Check sheet for the drawn part. Datum: minimum x, y, z corner. Units: mm. A direction names the side the tool comes from. Give positions to 0.01 mm unless a question says otherwise; leave off trailing zeros. Loops run counter-clockwise (first coordinate to the right, second up) from the corner with the lowest first, then second, coordinate; pieces in that order, holes last.
1. Cross-section at D-D, the plane x = 5.5. Record the cut outline in (y, z).
2. Material ranges on L1, parallel to X at y = 15.1, z = 1.5; L2, parallel to Y at x = 17, z = 4.25; L3, parallel to Z at x = 22, y = 15.25 (1 decimal), recorded low to high.
3. Tool access check on the marked faces 4, 5 and 6. Record the directions out of +Z, -Z, +X, -X, +Y, -Y that give a thin tool (end or side, any length) a straight path to the whole face; none if there is none.
4. Cross-section at B-B, the plane z = 1.5. Record the cut outline in (x, y).
5. Cross-section at A-A, the plane x = 23. Record the cut outline in (y, z).
6. Release check for a two-part mould opening along X. For the marked faces 1, 2 and 3 record: +X half, -X half, draft (parallel to the pull), parting line (faces both ways), or undercut.
7. Cross-section at C-C, the plane z = 7. Record the cut outline in (x, y).
8. Go/stop test with flat-tipped pins: pin 1 Ø3 at (x, y) = (10.5, 3.5) entering from -Z; pin 2 Ø4 at (x, z) = (19, 6.5) entering from -Y; pin 3 Ø3 at (y, z) = (3, 3) entering from -X. Record where each tip stops, or that it passes through.
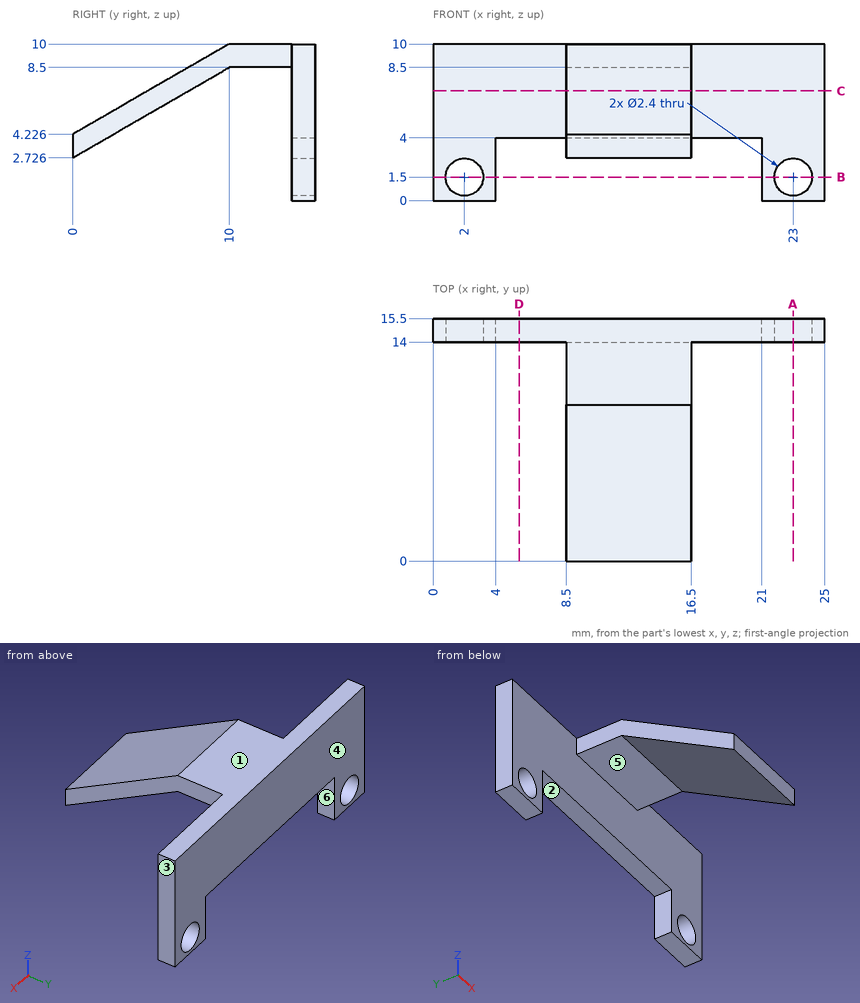
Result:
1. outline: (14, 4) - (15.5, 4) - (15.5, 10) - (14, 10) - close
2. L1: x = 0 to 0.8, 3.2 to 4, 21 to 21.8, 24.2 to 25
2. L2: y = 14 to 15.5
2. L3: z = 0 to 0.8, 2.2 to 10
3. face 4: +Z, -Z, +X, -X, +Y
3. face 5: -Z, +X, -X
3. face 6: -Z, +Y, -Y
4. outline: (0, 14) - (0.8, 14) - (0.8, 15.5) - (0, 15.5) - close; (3.2, 14) - (4, 14) - (4, 15.5) - (3.2, 15.5) - close; (21, 14) - (21.8, 14) - (21.8, 15.5) - (21, 15.5) - close; (24.2, 14) - (25, 14) - (25, 15.5) - (24.2, 15.5) - close
5. outline: (14, 0) - (15.5, 0) - (15.5, 0.3) - (14, 0.3) - close; (14, 2.7) - (15.5, 2.7) - (15.5, 10) - (14, 10) - close
6. face 1: draft
6. face 2: undercut
6. face 3: +X half
7. outline: (0, 14) - (25, 14) - (25, 15.5) - (0, 15.5) - close; (8.5, 4.8) - (16.5, 4.8) - (16.5, 7.4) - (8.5, 7.4) - close
8. pin 1: stops at z = 3.88
8. pin 2: stops at y = 14
8. pin 3: stops at x = 8.5
